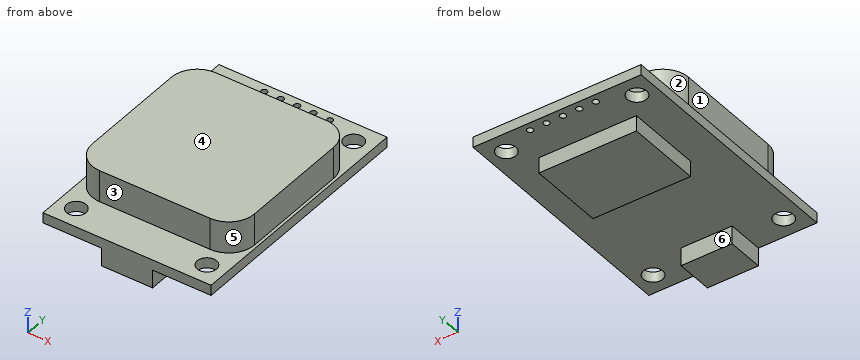
```python
from build123d import *

# Parameters (mm, degrees)
SKETCH_1_W                 = 26
SKETCH_1_H                 = 38
EXTRUDE_1_DEPTH            = 1.6
CUT_EXTRUDE_1_REACH        = 25.077
SKETCH_2_R                 = 1.5
SKETCH_3_W                 = 25.1
SKETCH_3_H                 = 25.1
EXTRUDE_2_DEPTH            = 4.9
FILLET_1_R                 = 4
SKETCH_6_W                 = 15.1
SKETCH_6_H                 = 11.7
EXTRUDE_3_DEPTH            = 2.4
SKETCH_7_W                 = 7.9
SKETCH_7_H                 = 5.7
EXTRUDE_4_DEPTH            = 2.8
CUT_EXTRUDE_2_REACH        = 25.922
SKETCH_8_R                 = 0.475
PATTERN_LINEAR_1_COUNT     = 3
PATTERN_LINEAR_1_PITCH     = 2.54
PATTERN_LINEAR_1_COL_COUNT = 3
PATTERN_LINEAR_1_COL_PITCH = 2.54


with BuildPart() as part:
    # 草图1 → 凸台-拉伸1 (new body)
    with BuildSketch(Plane.XY):
        Rectangle(SKETCH_1_W, SKETCH_1_H)
    extrude(amount=-EXTRUDE_1_DEPTH)

    # 草图2 → 切除-拉伸1 (cut, up to next)
    with BuildSketch(Plane.XY, mode=Mode.PRIVATE) as cut_extrude_1_sk1:
        with Locations((-10.1, 15.85)):
            Circle(SKETCH_2_R)
    cut_extrude_1_tool1 = extrude(cut_extrude_1_sk1.sketch, amount=-CUT_EXTRUDE_1_REACH, mode=Mode.PRIVATE) & part.part
    # 草图2 → 切除-拉伸1 (cut, up to next)
    with BuildSketch(Plane.XY, mode=Mode.PRIVATE) as cut_extrude_1_sk2:
        with Locations((10.1, 15.85)):
            Circle(SKETCH_2_R)
    cut_extrude_1_tool2 = extrude(cut_extrude_1_sk2.sketch, amount=-CUT_EXTRUDE_1_REACH, mode=Mode.PRIVATE) & part.part
    # 草图2 → 切除-拉伸1 (cut, up to next)
    with BuildSketch(Plane.XY, mode=Mode.PRIVATE) as cut_extrude_1_sk3:
        with Locations((10.1, -15.85)):
            Circle(SKETCH_2_R)
    cut_extrude_1_tool3 = extrude(cut_extrude_1_sk3.sketch, amount=-CUT_EXTRUDE_1_REACH, mode=Mode.PRIVATE) & part.part
    # 草图2 → 切除-拉伸1 (cut, up to next)
    with BuildSketch(Plane.XY, mode=Mode.PRIVATE) as cut_extrude_1_sk4:
        with Locations((-10.1, -15.85)):
            Circle(SKETCH_2_R)
    cut_extrude_1_tool4 = extrude(cut_extrude_1_sk4.sketch, amount=-CUT_EXTRUDE_1_REACH, mode=Mode.PRIVATE) & part.part
    add(cut_extrude_1_tool1.solids().sort_by_distance((-10.1, 15.85, 0))[0], mode=Mode.SUBTRACT)
    add(cut_extrude_1_tool2.solids().sort_by_distance((10.1, 15.85, 0))[0], mode=Mode.SUBTRACT)
    add(cut_extrude_1_tool3.solids().sort_by_distance((10.1, -15.85, 0))[0], mode=Mode.SUBTRACT)
    add(cut_extrude_1_tool4.solids().sort_by_distance((-10.1, -15.85, 0))[0], mode=Mode.SUBTRACT)

    # 草图3 → 凸台-拉伸2 (add)
    with BuildSketch(Plane.XY):
        with Locations((0, -0.44)):
            Rectangle(SKETCH_3_W, SKETCH_3_H)
    extrude(amount=EXTRUDE_2_DEPTH)

    # 圆角1
    fillet_1_edges = [part.edges().sort_by_distance(p)[0] for p in [
        (-12.55, 12.11, 2.45),
        (-12.55, -12.99, 2.45),
        (12.55, -12.99, 2.45),
        (12.55, 12.11, 2.45),
    ]]
    fillet(fillet_1_edges, radius=FILLET_1_R)

    # 草图6 → 凸台-拉伸3 (add)
    with BuildSketch(Plane(origin=(0, 0, -1.6), x_dir=(-1, 0, 0), z_dir=(0, 0, -1))):
        with Locations((0, 6.55)):
            Rectangle(SKETCH_6_W, SKETCH_6_H)
    extrude(amount=EXTRUDE_3_DEPTH)

    # 草图7 → 凸台-拉伸4 (add)
    with BuildSketch(Plane(origin=(0, 0, -1.6), x_dir=(-1, 0, 0), z_dir=(0, 0, -1))):
        with Locations((0, -16.15)):
            Rectangle(SKETCH_7_W, SKETCH_7_H)
    extrude(amount=EXTRUDE_4_DEPTH)

    # 草图8 → 切除-拉伸2 (cut, up to next)
    with BuildSketch(Plane(origin=(0, 0, -1.6), x_dir=(-1, 0, 0), z_dir=(0, 0, -1)), mode=Mode.PRIVATE) as cut_extrude_2_sk1:
        with Locations((0, 17.73)):
            Circle(SKETCH_8_R)
    cut_extrude_2_tool1 = extrude(cut_extrude_2_sk1.sketch, amount=-CUT_EXTRUDE_2_REACH, mode=Mode.PRIVATE) & part.part
    cut_extrude_2 = cut_extrude_2_tool1.solids().sort_by_distance((0, 17.73, -1.6))[0]
    add(cut_extrude_2, mode=Mode.SUBTRACT)

    # 阵列(线性)1: 切除-拉伸2 ×3
    with Locations(*[(-i * PATTERN_LINEAR_1_PITCH, 0, 0) for i in range(1, PATTERN_LINEAR_1_COUNT)]):
        add(cut_extrude_2, mode=Mode.SUBTRACT)

    # 阵列(线性)1 col: 切除-拉伸2 ×3
    with Locations(*[(i * PATTERN_LINEAR_1_COL_PITCH, 0, 0) for i in range(1, PATTERN_LINEAR_1_COL_COUNT)]):
        add(cut_extrude_2, mode=Mode.SUBTRACT)


solid = part.part
```
Here's how the part is built. I have some questions about the finished solid (model axes, mm). Face numbers are marked on the shaded views. A direction names the side the tool comes from. Coordinates: 2 decimals unless noted, no trailing zeros. Order: outer loops, then holes, each group sorted by start corner. A loop starts at its lowest first (then second) coordinate and runs counter-clockwise, first axis right, second up.
Item 1: Which directions (+Z, -Z, +X, -X, +Y, -Y) give clear straight access to the entire face, cutting with the end or side of a thin tool? Please do the marked faces 1, 2 and 3.
Response values:
face 1: +Z, -X, +Y, -Y
face 2: +Z, -X, +Y
face 3: +Z, +X, -X, -Y
Item 2: Thinking about a two-plate mould opening in Y: for the marked faces 4, 5 and 6, which applies, pulls with the +Y half, pulls with the -Y half, needs draft (parallel to the pull), parting line crosses it, or undercut?
Response values:
face 4: needs draft
face 5: pulls with the -Y half
face 6: undercut
Item 3: I need wall thicknesses on probe 1 along Y at (x, z) = (10.1, -0.65); probe 2 along Y at (x, z) = (-5.08, -1.05) (3 decimals); probe 3 along Z at (x, y) = (-2.75, 9). Which ranges of each line are inside material? Lowest first, please.
Response values:
probe 1: y = -19 to -17.35, -14.35 to 14.35, 17.35 to 19
probe 2: y = -19 to 17.255, 18.205 to 19
probe 3: z = -4 to 4.9
Item 4: If we section it at C-C, the plane x = 2.54: List the corners of the cut face in (y, z) for me (3 decimals), then the cut area to 3 significant figures.
Response values:
outline: (-19, -4.4) - (-13.3, -4.4) - (-13.3, -1.6) - (0.7, -1.6) - (0.7, -4) - (12.4, -4) - (12.4, -1.6) - (17.255, -1.6) - (17.255, 0) - (12.11, 0) - (12.11, 4.9) - (-12.99, 4.9) - (-12.99, 0) - (-19, 0) - close; (18.205, -1.6) - (19, -1.6) - (19, 0) - (18.205, 0) - close
area: 226 mm2
Item 5: I'm going to push flat-ended pins straight in: pin 1 Ø0.8 at (x, z) = (1.5, -3) entering from +Y; pin 2 Ø1.5 at (y, z) = (-3, 2) entering from -X; pin 3 Ø2.5 at (x, z) = (-3.5, 2) entering from +Y. Where does each tip first touch, or does it pass through?
Response values:
pin 1: stops at y = 12.4
pin 2: stops at x = -12.55
pin 3: stops at y = 12.11
Item 6: If we section it at A-A, the plane z = -3: List the corners of the cut face in (x, y) for me.
Response values:
outline: (-7.55, 0.7) - (7.55, 0.7) - (7.55, 12.4) - (-7.55, 12.4) - close; (-3.95, -19) - (3.95, -19) - (3.95, -13.3) - (-3.95, -13.3) - close
Item 7: If we section it at B-B, the plane y = 17.73: List the corners of the cut face in (x, z) for me (3 decimals), then the cut area to 3 significant figures.
Response values:
outline: (-13, -1.6) - (-5.555, -1.6) - (-5.555, 0) - (-13, 0) - close; (-4.605, -1.6) - (-3.015, -1.6) - (-3.015, 0) - (-4.605, 0) - close; (-2.065, -1.6) - (-0.475, -1.6) - (-0.475, 0) - (-2.065, 0) - close; (0.475, -1.6) - (2.065, -1.6) - (2.065, 0) - (0.475, 0) - close; (3.015, -1.6) - (4.605, -1.6) - (4.605, 0) - (3.015, 0) - close; (5.555, -1.6) - (13, -1.6) - (13, 0) - (5.555, 0) - close
area: 34.0 mm2
Item 8: If we section it at D-D, the plane z = -0.75: Give the number of separate pieces and of enclosed holes in the cut face, then the cut area to 3 significant figures.
Response values:
separate pieces: 1
enclosed holes: 9
area: 956 mm2
